Build history of the part. All positions in model axes, mm. Face numbers are marked on the shaded views. A direction names the side the tool comes from. Round coordinates to 2 decimals unless told otherwise and drop trailing zeros. Write each loop counter-clockwise with the first axis right and the second up, starting at its lowest first coordinate (ties: lowest second). Pieces come first, ordered by that corner, then holes. Notation, with made-up numbers: (89, 78) - (108, 78) arc R34 cw to (108, 117) - close; hole circle Ø8 at (-20.5, 63.25). An arc over 180 degrees is marked (long way). Write each question's results on one line, items separated by ' | '.
Autodesk Inventor part; units mm, degrees
ref_plane "Work Plane1" through (11.804, 0, 0) normal (0, 0, 1) x (-1, 0, 0)
ref_plane "YZ Plane" through (0, 0, 0) normal (1, 0, 0) x (0, 1, 0)
ref_plane "XZ Plane" through (0, 0, 0) normal (0, 1, 0) x (-1, 0, 0)
sketch "Sketch1" plane through (0, 0, 0) normal (1, 0, 0) x (0, 1, 0)
  line L0 (2.0207, -3.5) -> (-2.0207, -3.5)
  line L1 (-2.0207, -3.5) -> (-4.0415, 0)
  line L2 (-4.0415, 0) -> (-2.0207, 3.5)
  line L3 (-2.0207, 3.5) -> (2.0207, 3.5)
  line L4 (2.0207, 3.5) -> (4.0415, 0)
  line L5 (4.0415, 0) -> (2.0207, -3.5)
  point P0 (0, 0)
  point P1 (0, 0)
  dimension "d0" = 8.0829
extrude "Body" add sketch "Sketch1" along normal blind 3.2
sketch "Sketch2" plane through (3.2, 0, 0) normal (1, 0, 0) x (0, 0, -1)
  circle A0 centre (0, 0) radius 2.95
  dimension "d7" = 5.9
extrude "Ring" add sketch "Sketch2" along normal blind 1.8
sketch "Sketch3" plane through (0, 0, 0) normal (0, 0, 1) x (1, 0, 0)
  line L0 (0, 2.0207) -> (0, 4.0415)
  line L1 (0, 4.0415) -> (3.2, 4.0415)
  line L2 (3.2, 2.0207) -> (3.2, 4.0415)
  line L3 (-0.64, 0) -> (3.84, 0)
  line L4 (0, 2.95) -> (0.6302, 4.0415)
  line L5 (2.5698, 4.0415) -> (3.2, 2.95)
  dimension "d3" = 30
  dimension "d4" = 30
  dimension "d5" = 5.9
  dimension "d6" = 5.9
revolve "Chamfer1" cut sketch "Sketch3" angle 360 about axis through (-10, 0, 0) along (1, 0, 0)
sketch "Sketch4" plane through (0, 0, 0) normal (-1, 0, 0) x (0, 0, 1)
  line L0 (0, -5.658) -> (0, 5.658)
  line L1 (-4.9, 0) -> (4.9, 0)
  point P0 (0, 0)
hole "Thread" at (0, 0, 0) direction (1, 0, 0) diameter 3.242 end through all
chamfer "Chamfer2" distance 0.3789 angle 30 1 edges at (0, 0, -1.621) measured on face at (0, 2.4745, -0.3005)
chamfer "Chamfer3" distance 0.3789 angle 30 1 edges at (5, 0, -1.621) measured on face at (5, -0.3646, -2.4627)
ref_plane "Work Plane1" through (11.804, 0, 0) normal (0, 0, 1) x (-1, 0, 0)
equation "\"d0\" = 1.1547 * SW"
equation "\"d1\" = KOH1"
equation "\"d7\" = SD2"
equation "\"d8\" = KOH - KOH1"
equation "\"d3\" = ANG1"
equation "\"d4\" = ANG2"
equation "\"d5\" = SW0"
equation "\"d6\" = SW01"
equation "\"d10\" = -0.5 * GD1 + 0.5 * NND"
equation "\"d46\" = -0.5 * GD1 + 0.5 * NND"
equation "\"d12\" = -0.5 * GD1 + 0.5 * NND"
equation "\"d47\" = -0.5 * GD1 + 0.5 * NND"
equation "\"ANG1\" = 30deg"
equation "\"ANG2\" = 30deg"
equation "\"NND\" = 4"
equation "\"KOH1\" = 3.2"
equation "\"KOH\" = 5"
equation "\"SW\" = 7"
equation "\"SW0\" = 5.9"
equation "\"SW01\" = SW0"
equation "\"SD2\" = SW0"
equation "\"GUL\" = 0.541266 * PTC"
equation "\"THREADDIA\" = 4"
equation "\"TOA\" = 30deg"
equation "\"PTC\" = 0.7"
equation "\"E0\" = 1.155 * SW"
equation "\"GAL\" = 0.541266 * PTC"
properties part number "M4 - Nyloc Nut" material "Steel, Alloy"
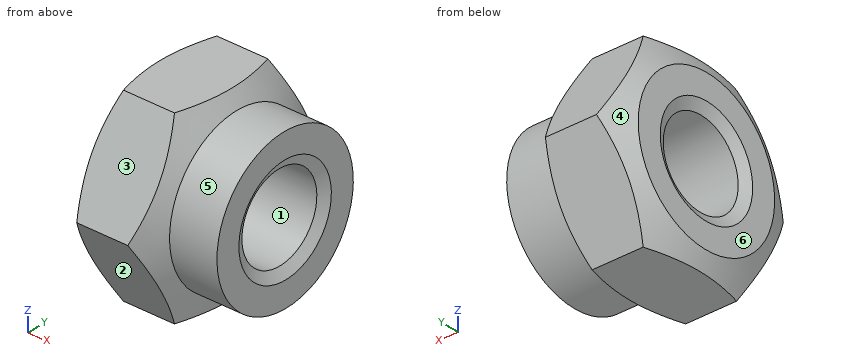
(1) Flat gauge pins, fed straight in: pin 1 Ø1.5 at (x, z) = (4, 1.5) entering from +Y; pin 2 Ø3.5 at (y, z) = (0, 0) entering from -X; pin 3 Ø1 at (x, z) = (3, 0) entering from -Y. Where does each tip first touch, or does it go through?
Worked answers:
pin 1: stops at y = 2.85 | pin 2: stops at x = 0.14 | pin 3: stops at y = -4.04
(2) Tool access for the marked faces 5 and 6: list every direction of +Z, -Z, +X, -X, +Y, -Y with a clear straight run to the whole face (end or side of a thin tool).
Worked answers:
face 5: +X | face 6: +Z, -Z, -X, +Y, -Y
(3) Slice it at B-B, the plane x = 3.45. Write the cut outline in (y, z), and give its area (3 significant figures).
Worked answers:
outline: circle Ø5.9 at (0, 0); hole circle Ø3.24 at (0, 0) | area: 19.1 mm2
(4) Slice it at A-A, the plane y = 0. Write the cut outline in (x, z).
Worked answers:
outline: (0, -2.95) - (0.32, -3.5) - (2.88, -3.5) - (3.2, -2.95) - (5, -2.95) - (5, -2) - (4.78, -1.62) - (0.22, -1.62) - (0, -2) - close; (0, 2) - (0.22, 1.62) - (4.78, 1.62) - (5, 2) - (5, 2.95) - (3.2, 2.95) - (2.88, 3.5) - (0.32, 3.5) - (0, 2.95) - close
(5) Two-plate mould, pull along Z, no slides. Class the marked faces 1, 2, 3 and 4: released by +Z, released by -Z, zero draft, split by the parting line, or undercut.
Worked answers:
face 1: undercut | face 2: released by -Z | face 3: released by +Z | face 4: split by the parting line
(6) Drill centre lines: probe 1 along Z at (x, y) = (2.15, 0); probe 2 along Z at (x, y) = (3.5, 0); probe 3 along Y at (x, z) = (1.45, -1). Where is each one in solid material? Low to high. Write a range as [from, to].
Worked answers:
probe 1: z = [-3.5, -1.62], [1.62, 3.5] | probe 2: z = [-2.95, -1.62], [1.62, 2.95] | probe 3: y = [-3.46, -1.28], [1.28, 3.46]
